Autodesk Inventor part; units mm, degrees
ref_plane "YZ Plane" through (0, 0, 0) normal (1, 0, 0) x (0, 1, 0)
ref_plane "XZ Plane" through (0, 0, 0) normal (0, 1, 0) x (-1, 0, 0)
ref_plane "XY Plane" through (0, 0, 0) normal (0, 0, 1) x (1, 0, 0)
sketch "Boceto1" plane through (0, 0, 0) normal (0, 0, 1) x (1, 0, 0)
  line L0 (0, 0) -> (30, 0)
  line L1 (30, 0) -> (30, 60)
  line L2 (30, 60) -> (0, 60)
  line L3 (0, 60) -> (0, 0)
  circle A0 centre (15, 30) radius 4.25
  circle A1 centre (7, 30) radius 1
  circle A2 centre (23, 30) radius 1
  circle A3 centre (15, 37) radius 1
  circle A4 centre (15, 21) radius 1
  circle A5 centre (15, 50) radius 2
  circle A6 centre (15, 10) radius 2
  point P0 (15, 0)
  dimension "d0" = 30
  dimension "d1" = 60
  dimension "d2" = 8.5
  dimension "d3" = 2
  dimension "d4" = 2
  dimension "d7" = 2
  dimension "d8" = 2
  dimension "d9" = 16
  dimension "d21" = 30
  dimension "d22" = 23
  dimension "d24" = 0
  dimension "d25" = 0
  dimension "d26" = 16
  dimension "d27" = 7
  dimension "d28" = 4
  dimension "d29" = 4
  dimension "d30" = 20
  dimension "d31" = 20
extrude "Extrusión1" add sketch "Boceto1" along normal blind 3
thread "Rosca1"
thread "Rosca2"
thread "Rosca3"
thread "Rosca4"
thread "Rosca5"
thread "Rosca6"
sketch "Boceto2" plane through (0, 0, 3) normal (0, 0, 1) x (1, 0, 0)
  line L0 (30, 60) -> (0, 60)
  line L1 (0, 60) -> (8, 60)
  line L2 (8, 60) -> (8, 45)
  line L3 (8, 45) -> (0, 45)
  line L4 (0, 45) -> (0, 60)
  line L5 (30, 60) -> (22, 60)
  line L6 (22, 60) -> (22, 45)
  line L7 (22, 45) -> (30, 45)
  line L8 (30, 45) -> (30, 60)
  line L9 (0, 0) -> (30, 0)
  line L10 (0, 0) -> (8, 0)
  line L11 (8, 0) -> (8, 15)
  line L12 (8, 15) -> (0, 15)
  line L13 (0, 15) -> (0, 0)
  line L14 (30, 0) -> (22, 0)
  line L15 (22, 0) -> (22, 15)
  line L16 (22, 15) -> (30, 15)
  line L17 (30, 15) -> (30, 0)
  dimension "d36" = 8
  dimension "d37" = 15
  dimension "d38" = 8
  dimension "d39" = 15
  dimension "d40" = 8
  dimension "d41" = 15
  dimension "d42" = 8
  dimension "d43" = 15
extrude "Extrusión2" cut sketch "Boceto2" against normal blind 3
properties part number "placa_soporte_motor"
Model file for the job. Use its own axes, mm. A direction names the side the tool comes from. Coordinates: 2 decimals unless noted, no trailing zeros. Write each loop counter-clockwise with the first axis right and the second up, starting at its lowest first coordinate (ties: lowest second). Pieces come first, ordered by that corner, then holes. Notation, with made-up numbers: (28, 75.5) - (50, 75.5) arc R23 cw to (50, 108.5) - close; hole circle Ø8 at (-40, 30.25). An arc over 180 degrees is marked (long way). One line per item, written item: value. Start each with the question number.
1. Tool access for faces 4 (the flat face through (22, 53, 2)), 5 (the flat face through (8, 53, 2)), 6 (the flat face through (8, 7, 2)), 7 (the cylindrical face through (11.63, 32.59, 1.48)): list every direction of +Z, -Z, +X, -X, +Y, -Y with a clear straight run to the whole face (end or side of a thin tool).
2. Slice it at D-D (z = 1.3). Write the cut outline in (x, y), plus the area to 3 significant figures.
3. Probe line 1 (Y direction, x = 15, z = 1.6); line 2 (Y direction, x = 23, z = 1.45); line 3 (X direction, y = 7, z = 1.1). List the from-to ranges inside material, lowest first. Write a range as from..to.
4. Slice it at B-B (y = 21). Write the cut outline in (x, z).
5. Slice it at A-A (x = 15). Write the cut outline in (y, z).
6. Slice it at C-C (x = 23). Write the cut outline in (y, z), plus the area to 3 significant figures.
7. Mould opens along X. For faces 1 (the cylindrical face through (7, 29, 1)), 2 (the flat face through (26, 15, 2)), 3 (the flat face through (22, 7, 2)) say: released by +X, released by -X, zero draft, split by the parting line, or undercut.
8. Flat gauge pins, fed straight in: pin 1 (1.5 mm diameter, centred on y = 56, z = 2, fed in from +X); pin 2 (7 mm diameter, centred on x = 15, y = 30, fed in from -Z); pin 3 (1.5 mm diameter, centred on y = 54, z = 1.5, fed in from -X). Where does each tip first touch, or does it go through?
Answers below:
1. face 4: +Z, -Z, +X, +Y
1. face 5: +Z, -Z, -X, +Y
1. face 6: +Z, -Z, -X, -Y
1. face 7: +Z, -Z
2. outline: (0, 15) - (8, 15) - (8, 0) - (22, 0) - (22, 15) - (30, 15) - (30, 45) - (22, 45) - (22, 60) - (8, 60) - (8, 45) - (0, 45) - close; hole circle Ø2 at (7, 30); hole circle Ø8.5 at (15, 30); hole circle Ø4 at (15, 10); hole circle Ø4 at (15, 50); hole circle Ø2 at (15, 21); hole circle Ø2 at (15, 37); hole circle Ø2 at (23, 30)
2. area: 1,230 mm^2
3. line 1: y = 0..8, 12..20, 22..25.75, 34.25..36, 38..48, 52..60
3. line 2: y = 15..29, 31..45
3. line 3: x = 8..22
4. outline: (0, 0) - (14, 0) - (14, 3) - (0, 3) - close; (16, 0) - (30, 0) - (30, 3) - (16, 3) - close
5. outline: (0, 0) - (8, 0) - (8, 3) - (0, 3) - close; (12, 0) - (20, 0) - (20, 3) - (12, 3) - close; (22, 0) - (25.75, 0) - (25.75, 3) - (22, 3) - close; (34.25, 0) - (36, 0) - (36, 3) - (34.25, 3) - close; (38, 0) - (48, 0) - (48, 3) - (38, 3) - close; (52, 0) - (60, 0) - (60, 3) - (52, 3) - close
6. outline: (15, 0) - (29, 0) - (29, 3) - (15, 3) - close; (31, 0) - (45, 0) - (45, 3) - (31, 3) - close
6. area: 84.0 mm^2
7. face 1: undercut
7. face 2: zero draft
7. face 3: released by +X
8. pin 1: stops at x = 22
8. pin 2: passes through
8. pin 3: stops at x = 8
